CAD build for the part. Positions are in the model's coordinates, mm. Face numbers are marked on the shaded views. A direction names the side the tool comes from. Round coordinates to 2 decimals unless told otherwise and drop trailing zeros. Order: outer loops, then holes, each group sorted by start corner. A loop starts at its lowest first (then second) coordinate and runs counter-clockwise, first axis right, second up. Notation, with made-up numbers: (4.25, 1.25) - (26.25, 1.25) arc R14 cw to (26.25, 24.25) - close; hole circle Ø2 at (29.25, -3). An arc over 180 degrees is marked (long way). Use one line per item in the form item = value. Start each with the question number.
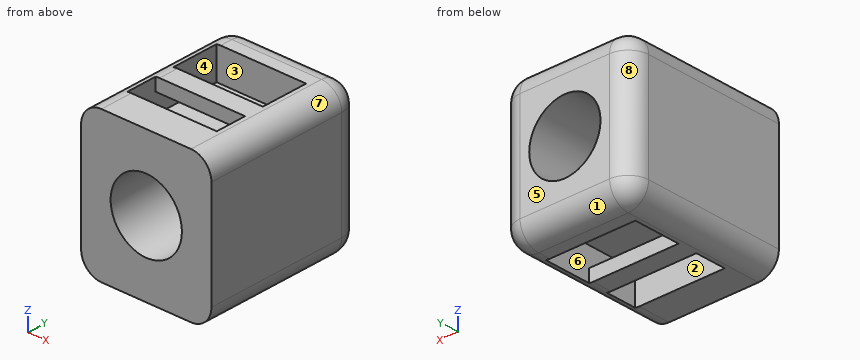
Autodesk Inventor part; units mm, degrees
ref_plane "YZ Plane" through (0, 0, 0) normal (1, 0, 0) x (0, 1, 0)
ref_plane "XZ Plane" through (0, 0, 0) normal (0, 1, 0) x (-1, 0, 0)
ref_plane "XY Plane" through (0, 0, 0) normal (0, 0, 1) x (1, 0, 0)
sketch "Sketch1" plane through (0, 0, 0) normal (0, 1, 0) x (-1, 0, 0)
  line L0 (-9.525, -8.255) -> (10.795, -8.255)
  line L1 (10.795, -8.255) -> (10.795, 14.605)
  line L2 (10.795, 14.605) -> (-9.525, 14.605)
  line L3 (-9.525, 14.605) -> (-9.525, -8.255)
  line L4 (-9.525, -8.255) -> (10.795, 14.605) construction
  line L5 (10.795, -8.255) -> (-9.525, 14.605) construction
  point P0 (0.635, 3.175)
  dimension "d9" = 20.32
  dimension "d10" = 22.86
extrude "Extrusion3" add sketch "Sketch1" along normal blind 25.4
sketch "actual_circle" plane through (0, 25.4, 0) normal (0, 1, 0) x (1, 0, 0)
  circle A0 centre (-0.635, -3.175) radius 5.5563
  line L0 (9.525, 8.255) -> (-10.795, 8.255)
  line L1 (-10.795, 8.255) -> (-10.795, -14.605)
  dimension "d27" = 11.1125
  dimension "d57" = 11.43
  dimension "d58" = 10.16
extrude "Extrusion6" cut sketch "actual_circle" against normal blind 50.8
sketch "circle" plane through (-10.795, 0, 14.605) normal (0, 0, 1) x (1, 0, 0)
  line L0 (2.54, 20.32) -> (16.51, 20.32)
  line L1 (16.51, 20.32) -> (16.51, 5.08)
  line L2 (16.51, 5.08) -> (2.54, 5.08)
  line L3 (2.54, 5.08) -> (2.54, 20.32)
  line L4 (0, 25.4) -> (20.32, 25.4)
  line L5 (0, 0) -> (0, 25.4)
  point P0 (10.795, 0)
  dimension "d32" = 13.97
  dimension "d33" = 15.24
  dimension "d34" = 5.08
  dimension "d35" = 2.54
extrude "Extrusion7" cut sketch "circle" against normal blind 5.08
sketch "Sketch7" plane through (9.525, 0, -8.255) normal (0, 0, -1) x (-1, 0, 0)
  line L0 (2.54, 20.32) -> (16.51, 20.32)
  line L1 (16.51, 20.32) -> (16.51, 5.08)
  line L2 (16.51, 5.08) -> (2.54, 5.08)
  line L3 (2.54, 5.08) -> (2.54, 20.32)
  line L4 (0, 0) -> (0, 25.4)
  line L5 (0, 25.4) -> (20.32, 25.4)
  point P0 (9.525, 0)
  dimension "d38" = 13.97
  dimension "d39" = 15.24
  dimension "d40" = 2.54
  dimension "d41" = 5.08
extrude "Extrusion8" cut sketch "Sketch7" against normal blind 5.08
sketch "Lock" plane through (-6.985, 5.08, -8.255) normal (1, 0, 0) x (0, 0, -1)
  line L0 (-2.032, 7.874) -> (0, 7.874)
  line L1 (0, 7.874) -> (0, 4.826)
  line L2 (0, 4.826) -> (-2.032, 4.826)
  line L3 (-2.032, 4.826) -> (-2.032, 7.874)
  line L4 (-5.08, 15.24) -> (-5.08, 0)
  line L5 (0, 15.24) -> (0, 0)
  point P0 (-8.255, -5.08)
  dimension "d44" = 2.032
  dimension "d45" = 3.048
  dimension "d46" = 7.366
  dimension "d59" = 0
extrude "Extrusion9" add sketch "Lock" along normal blind 13.97
sketch "Sketch9" plane through (-8.255, 5.08, 14.605) normal (1, 0, 0) x (0, 0, -1)
  line L0 (0, 7.874) -> (2.032, 7.874)
  line L1 (2.032, 7.874) -> (2.032, 4.826)
  line L2 (2.032, 4.826) -> (0, 4.826)
  line L3 (0, 4.826) -> (0, 7.874)
  line L4 (0, 0) -> (0, 15.24)
  point P0 (14.605, -5.08)
  dimension "d50" = 2.032
  dimension "d51" = 3.048
  dimension "d52" = 0
  dimension "d53" = 7.366
extrude "Extrusion10" add sketch "Sketch9" along normal blind 13.97
fillet "Fillet1" radius 3.175 4 edges at (-10.795, 25.4, 3.175) (9.525, 25.4, 3.175) (-0.635, 25.4, 14.605) (-0.635, 25.4, -8.255)
fillet "Fillet2" radius 3.175 8 edges at (8.5951, 24.4701, 13.6751) (9.525, 11.1125, 14.605) (8.5951, 24.4701, -7.3251) (9.525, 11.1125, -8.255) (-9.8651, 24.4701, -7.3251) (-10.795, 11.1125, -8.255) (-9.8651, 24.4701, 13.6751) (-10.795, 11.1125, 14.605)
properties part number "TM_Weird_Box_LMMM"
(1) Slice it at C-C (y = 10.5). Give the cut face in (x, z) (3 decimals), and give its area (3 significant figures).
(2) Slice it at A-A (z = 4.5). Give the cut face in (x, y) (3 decimals).
(3) Slice it at D-D (y = 18.25). Give the cut face in (x, z) (3 decimals).
(4) Which spindle directions (+Z, -Z, +X, -X, +Y, -Y) get a long thin tool onto all of the face, cutting with end or side? Do the marked faces 1, 2, 3, 4 and 5. Say none if no direction does.
(5) Wall check: line 1 (Y direction, x = 3.75, z = 11.5); line 2 (X direction, y = 15.5, z = 3) (3 decimals); line 3 (X direction, y = 15.25, z = 10.75) (3 decimals). Give the ranges that are in metal, low to high. Write a range as [from, to].
(6) Slice it at B-B (x = -1.25). Give the cut face in (y, z) (3 decimals).
(7) Mould opens along X. For the marked faces 6, 7 and 8 say: pulls with the +X half, pulls with the -X half, needs draft (parallel to the pull), parting line crosses it, or undercut.
(8) Flat gauge pins, fed straight in: P1, Ø1.5, axis at y = 9.5, z = 13.5, coming from the -X side; P2, Ø1, axis at x = -3.5, z = 14, coming from the +Y side. Where does each tip first touch, or does it go through?
Results list:
q1.outline = (-10.795, -5.08) arc R3.175 ccw to (-7.62, -8.255) - (6.35, -8.255) arc R3.175 ccw to (9.525, -5.08) - (9.525, 11.43) arc R3.175 ccw to (6.35, 14.605) - (-7.62, 14.605) arc R3.175 ccw to (-10.795, 11.43) - close; hole (-8.255, 9.525) - (5.715, 9.525) - (5.715, 12.573) - (-8.255, 12.573) - close; hole (-6.985, -6.223) - (6.985, -6.223) - (6.985, -3.175) - (-6.985, -3.175) - close; hole circle Ø11.113 at (-0.635, 3.175)
q1.area = 274 mm²
q2.outline = (-10.795, 0) - (-6.031, 0) - (-6.031, 25.4) - (-7.62, 25.4) arc R3.175 ccw to (-10.795, 22.225) - close; (4.761, 0) - (9.525, 0) - (9.525, 22.225) arc R3.175 ccw to (6.35, 25.4) - (4.761, 25.4) - close
q3.outline = (-10.795, -5.08) arc R3.175 ccw to (-7.62, -8.255) - (-6.985, -8.255) - (-6.985, -3.175) - (6.985, -3.175) - (6.985, -8.191) arc R3.175 ccw to (9.525, -5.08) - (9.525, 11.43) arc R3.175 ccw to (6.35, 14.605) - (5.715, 14.605) - (5.715, 9.525) - (-8.255, 9.525) - (-8.255, 14.541) arc R3.175 ccw to (-10.795, 11.43) - close; hole circle Ø11.113 at (-0.635, 3.175)
q4.face_1 = -Z, +X, -X, +Y
q4.face_2 = -Z
q4.face_3 = +Z
q4.face_4 = none
q4.face_5 = +Z, -Z, +X, -X, +Y
q5.line_1 = [0, 5.08], [20.32, 25.4]
q5.line_2 = [-10.795, -6.189], [4.919, 9.525]
q5.line_3 = [-10.795, -8.255], [5.715, 9.525]
q6.outline = (0, -8.255) - (5.08, -8.255) - (5.08, -3.175) - (20.32, -3.175) - (20.32, -8.255) - (22.225, -8.255) arc R3.175 ccw to (25.4, -5.08) - (25.4, -2.347) - (0, -2.347) - close; (0, 8.697) - (25.4, 8.697) - (25.4, 11.43) arc R3.175 ccw to (22.225, 14.605) - (20.32, 14.605) - (20.32, 9.525) - (5.08, 9.525) - (5.08, 14.605) - (0, 14.605) - close; (9.906, -8.255) - (12.954, -8.255) - (12.954, -6.223) - (9.906, -6.223) - close; (9.906, 12.573) - (12.954, 12.573) - (12.954, 14.605) - (9.906, 14.605) - close
q7.face_6 = undercut
q7.face_7 = pulls with the +X half
q7.face_8 = pulls with the -X half
q8.P1 = -10.51
q8.P2 = 24.63
